Input: part model. Units: mm. Frame: model coordinates. A direction names the side the tool comes from. Round coordinates to 2 decimals unless told otherwise and drop trailing zeros. Write each loop counter-clockwise with the first axis right and the second up, starting at its lowest first coordinate (ties: lowest second). Pieces come first, ordered by that corner, then holes. Notation, with made-up numbers: (18.25, 9.25) -> (31.25, 9.25) arc R29 cw to (31.25, 45.25) -> close; hole circle Ø11 at (4, 61.25). An arc over 180 degrees is marked (long way). Use CSV: the item, a comma, the result in double quotes.
```python
from build123d import *

# Parameters (mm, degrees)
F0_W      = 20.574
F0_H      = 20.574
F1_DEPTH  = 7.112
F2_W      = 17.018
F2_H      = 17.018
F3_DEPTH  = 5.334
F4_R      = 2.54
F5_W      = 5.588
F5_H      = 12.7
F6_DEPTH  = 3.048
F7_W      = 11.176
F7_H      = 12.7
F8_DEPTH  = 3.048
F9_W      = 4.064
F9_H      = 9.906
F10_DEPTH = 1.778
F11_R     = 1.27
F12_R     = 1.27


with BuildPart() as f1:
    # F0 (on Top) → F1 (new body)
    with BuildSketch(Plane.XY):
        Rectangle(F0_W, F0_H)
    extrude(amount=F1_DEPTH)

    # F2 (on face) → F3 (cut)
    with BuildSketch(Plane(origin=(0, 0, 0), x_dir=(1, 0, 0), z_dir=(0, 0, -1))):
        Rectangle(F2_W, F2_H)
    extrude(amount=-F3_DEPTH, mode=Mode.SUBTRACT)

    # F4
    f4_edges = [f1.edges().sort_by_distance(p)[0] for p in [
        (-10.287, -10.287, 3.556),
        (10.287, 10.287, 3.556),
        (10.287, -10.287, 3.556),
        (-10.287, 10.287, 3.556),
    ]]
    fillet(f4_edges, radius=F4_R)

    # F5 (on face) → F6 (cut)
    with BuildSketch(Plane.XY.offset(7.112)):
        with Locations((-7.493, 0)):
            Rectangle(F5_W, F5_H)
    extrude(amount=-F6_DEPTH, mode=Mode.SUBTRACT)

    # F7 (on face) → F8 (cut)
    with BuildSketch(Plane.XY.offset(7.112)):
        with Locations((10.287, 0)):
            Rectangle(F7_W, F7_H)
    extrude(amount=-F8_DEPTH, mode=Mode.SUBTRACT)

    # F9 (on face) → F10 (cut)
    with BuildSketch(Plane.XY.offset(7.112)):
        Rectangle(F9_W, F9_H)
    extrude(amount=-F10_DEPTH, mode=Mode.SUBTRACT)

    # F11
    f11_edges = [f1.edges().sort_by_distance(p)[0] for p in [
        (0, 10.287, 7.112),
        (0, -10.287, 7.112),
    ]]
    fillet(f11_edges, radius=F11_R)

    # F12
    f12_edges = [f1.edges().sort_by_distance(p)[0] for p in [
        (-10.287, 0, 0),
        (0, 10.287, 0),
        (-9.543051, 9.543051, 0),
    ]]
    fillet(f12_edges, radius=F12_R)


solid = f1.part
```
Item 1: Section query C-C on y = 3.25. Return the cut outline in (x, z).
Worked answers:
outline,"(-10.29, 1.27) arc R1.27 ccw to (-9.02, 0) -> (-8.51, 0) -> (-8.51, 4.06) -> (-10.29, 4.06) -> close; (-4.7, 5.33) -> (-2.03, 5.33) -> (-2.03, 7.11) -> (-4.7, 7.11) -> close; (2.03, 5.33) -> (4.7, 5.33) -> (4.7, 7.11) -> (2.03, 7.11) -> close; (8.51, 0) -> (9.02, 0) arc R1.27 ccw to (10.29, 1.27) -> (10.29, 4.06) -> (8.51, 4.06) -> close"
Item 2: Pull-direction query (X, two-part tool) for faces 4 (the face through (0, 4.953, 6)), 5 (the face through (9.905, -7.039, 6.75)), 6 (the face through (-4.699, 0, 6)); classes: +X half, -X half, draft (parallel to the pull), parting line (faces both ways), or undercut.
Worked answers:
face 4,"undercut"
face 5,"+X half"
face 6,"-X half"
Item 3: Set-up query: faces 1 (the face through (0, -4.953, 6)), 2 (the face through (-9, 0, 4.064)), 3 (the face through (0, 8.509, 3)). Return all of +Z, -Z, +X, -X, +Y, -Y with unobstructed straight access to the full face (end or side cutting, diameter ignored); none if empty.
Worked answers:
face 1,"+Z, -Z"
face 2,"+Z, +X, -X"
face 3,"-Z"
Item 4: First-contact query: pin 1 Ø5 at (x, y) = (-4, -1) entering from -Z; pin 2 Ø1.4 at (y, z) = (-0.5, 6) entering from -X; pin 3 Ø0.5 at (x, z) = (0.5, 6.5) entering from -Y. Flat tips, straight axial feed; report the tip coordinate or a pass-through.
Worked answers:
pin 1,"stops at z = 5.33"
pin 2,"stops at x = -4.7"
pin 3,"stops at y = -10.22"
Item 5: Section query B-B on z = 5. Return the cut outline in (x, y).
Worked answers:
outline,"(-10.29, -7.75) arc R2.54 ccw to (-7.75, -10.29) -> (7.75, -10.29) arc R2.54 ccw to (10.29, -7.75) -> (10.29, -6.35) -> (8.51, -6.35) -> (8.51, -8.51) -> (-8.51, -8.51) -> (-8.51, -6.35) -> (-10.29, -6.35) -> close; (-10.29, 6.35) -> (-8.51, 6.35) -> (-8.51, 8.51) -> (8.51, 8.51) -> (8.51, 6.35) -> (10.29, 6.35) -> (10.29, 7.75) arc R2.54 ccw to (7.75, 10.29) -> (-7.75, 10.29) arc R2.54 ccw to (-10.29, 7.75) -> close"
Item 6: Section query D-D on z = 2.75. Return the cut outline in (x, y).
Worked answers:
outline,"(-10.29, -7.75) arc R2.54 ccw to (-7.75, -10.29) -> (7.75, -10.29) arc R2.54 ccw to (10.29, -7.75) -> (10.29, 7.75) arc R2.54 ccw to (7.75, 10.29) -> (-7.75, 10.29) arc R2.54 ccw to (-10.29, 7.75) -> close; hole (-8.51, -8.51) -> (8.51, -8.51) -> (8.51, 8.51) -> (-8.51, 8.51) -> close"
Item 7: Line query: line 1 (Y direction, x = 2.5, z = 1.5); line 2 (X direction, y = 4.5, z = 6.5). Output: solid intervals per line, ascending.
Worked answers:
line 1,"y = -10.29 to -8.51, 8.51 to 10.29"
line 2,"x = -4.7 to -2.03, 2.03 to 4.7"
Item 8: Section query A-A on x = -0.5. Return the cut outline in (y, z), plus the area to 3 significant figures.
Worked answers:
outline,"(-10.29, 1.27) arc R1.27 ccw to (-9.02, 0) -> (-8.51, 0) -> (-8.51, 5.33) -> (-4.95, 5.33) -> (-4.95, 7.11) -> (-9.02, 7.11) arc R1.27 ccw to (-10.29, 5.84) -> close; (4.95, 5.33) -> (8.51, 5.33) -> (8.51, 0) -> (9.02, 0) arc R1.27 ccw to (10.29, 1.27) -> (10.29, 5.84) arc R1.27 ccw to (9.02, 7.11) -> (4.95, 7.11) -> close"
area,"36.6 mm²"
